Read the model definition and answer for the solid it produces. Units are mm, in the model's axes. A direction names the side the tool comes from. Coordinates: 2 decimals unless noted, no trailing zeros. Order: outer loops, then holes, each group sorted by start corner. A loop starts at its lowest first (then second) coordinate and runs counter-clockwise, first axis right, second up.
```python
from build123d import *

# Parameters (mm, degrees)
F0_R     = 40
F1_DEPTH = 30
F2_W     = 15
F2_H     = 25
F3_DEPTH = 25
F4_R     = 5
F5_DEPTH = 61.901644


with BuildPart() as f1:
    # F0 (on Front) → F1 (new body)
    with BuildSketch(Plane.XZ):
        Circle(F0_R)
    extrude(amount=-F1_DEPTH)

    # F2 (on face) → F3 (cut)
    with BuildSketch(Plane(origin=(0, 30, 0), x_dir=(-1, 0, 0), z_dir=(0, 1, 0))):
        Rectangle(F2_W, F2_H)
    extrude(amount=-F3_DEPTH, mode=Mode.SUBTRACT)

    # F4 (on face) → F5 (cut, symmetric)
    with BuildSketch(Plane.YZ.offset(-7.5)):
        with Locations((17.5, 0)):
            Circle(F4_R)
    extrude(amount=F5_DEPTH, both=True, mode=Mode.SUBTRACT)


solid = f1.part
```
1) A cutting plane is placed at C-C, the plane y = 26.5. Determine the outline of the cut face in (x, z), and give its area (3 significant figures).
A:
outline: circle Ø80 at (0, 0); hole (-7.5, -12.5) - (7.5, -12.5) - (7.5, 12.5) - (-7.5, 12.5) - close
area: 4,650 mm2
2) A cutting plane is placed at B-B, the plane y = 15. Determine the outline of the cut face in (x, z), and give its area (3 significant figures).
A:
outline: (-39.76, -4.33) arc R40 ccw to (39.76, -4.33) - (7.5, -4.33) - (7.5, -12.5) - (-7.5, -12.5) - (-7.5, -4.33) - close; (-39.76, 4.33) - (-7.5, 4.33) - (-7.5, 12.5) - (7.5, 12.5) - (7.5, 4.33) - (39.76, 4.33) arc R40 ccw to start
area: 4,090 mm2
3) Which of the six approach directions +Z, -Z, +X, -X, +Y, -Y give full straight-line access (tool end or side, diameter ignored) to faces 5 (the cylindrical face through (23.978, 12.505, 0.22)), 6 (the flat face through (-7.5, 23, 0))?
A:
face 5: +X, -X
face 6: +Y
4) A cutting plane is placed at D-D, the plane x = 0. Determine the outline of the cut face in (y, z).
A:
outline: (0, -40) - (30, -40) - (30, -12.5) - (5, -12.5) - (5, 12.5) - (30, 12.5) - (30, 40) - (0, 40) - close
5) Determine the mould class of faces 1 (the flat face through (0, 18, 12.5)), 2 (the flat face through (0, 18, -12.5)), 3 (the flat face through (-1, 0, 1)), 4 (the cylindrical face through (38.153, 14.79, 12.015)) for opening direction Z: pulls with the +Z half, pulls with the -Z half, needs draft (parallel to the pull), parting line crosses it, or undercut.
A:
face 1: undercut
face 2: undercut
face 3: needs draft
face 4: parting line crosses it
6) Straight lines are drawn through the part: line 1 (Y direction, x = 15, z = 0); line 2 (Z direction, x = -1, y = 12); line 3 (X direction, y = 9.5, z = 0). For each, find the intervals that lie inside material, in ascending order.
A:
line 1: y = 0 to 12.5, 22.5 to 30
line 2: z = -39.99 to -12.5, 12.5 to 39.99
line 3: x = -40 to -7.5, 7.5 to 40
7) A cutting plane is placed at A-A, the plane z = 0. Determine the outline of the cut face in (x, y).
A:
outline: (-40, 0) - (40, 0) - (40, 12.5) - (7.5, 12.5) - (7.5, 5) - (-7.5, 5) - (-7.5, 12.5) - (-40, 12.5) - close; (-40, 22.5) - (-7.5, 22.5) - (-7.5, 30) - (-40, 30) - close; (7.5, 22.5) - (40, 22.5) - (40, 30) - (7.5, 30) - close
8) Flat-ended cylindrical pins translate along their axes: pin 1 Ø4.5 at (x, y) = (3.5, 20.5) entering from -Z; pin 2 Ø6 at (y, z) = (17.5, 0) entering from +X; pin 3 Ø4.5 at (x, y) = (-1.5, 23.5) entering from +Z; pin 4 Ø8 at (y, z) = (13.5, 18.5) entering from -X. Find the tip coordinate at first contact, or state that the pin passes through.
A:
pin 1: stops at z = -39.98
pin 2: passes through
pin 3: stops at z = 40
pin 4: stops at x = -37.28
